Check sheet for the modelled part. Datum: model origin and axes. Units: mm. A direction names the side the tool comes from. Give positions to 0.01 mm unless a question says otherwise; leave off trailing zeros. Write each loop counter-clockwise with the first axis right and the second up, starting at its lowest first coordinate (ties: lowest second). Pieces come first, ordered by that corner, then holes. Notation, with made-up numbers: (65.5, 20.5) -> (79.5, 20.5) arc R16 cw to (79.5, 37.5) -> close; hole circle Ø9 at (75, 1). An arc over 180 degrees is marked (long way). Answer as a JSON object with one key per item and string values.
from build123d import *

# Parameters (mm, degrees)
SKETCH1_W           = 22
SKETCH1_H           = 11
BOSS_EXTRUDE1_DEPTH = 24
BOSS_EXTRUDE2_DEPTH = 4
SKETCH4_W           = 11
SKETCH4_H           = 2
BOSS_EXTRUDE3_DEPTH = 3
SKETCH5_R           = 1
CUT_EXTRUDE2_DEPTH  = 21
SKETCH3_R           = 2.25
BOSS_EXTRUDE4_DEPTH = 3


with BuildPart() as part:
    # Sketch1 → Boss-Extrude1 (new body)
    with BuildSketch(Plane(origin=(0, 0, 0), x_dir=(1, 0, 0), z_dir=(0, 1, 0))):
        Rectangle(SKETCH1_W, SKETCH1_H)
    extrude(amount=BOSS_EXTRUDE1_DEPTH)

    # Sketch2 → Boss-Extrude2 (add)
    with BuildSketch(Plane(origin=(0, 24, 0), x_dir=(1, 0, 0), z_dir=(0, 1, 0))):
        with BuildLine():
            Line((-0.5, 2.006506876), (0.376524617, 2.006506876))
            ThreePointArc((0.376524617, 2.006506876), (11, 0.006506876), (0.376524617, -1.993493124))
            Line((0.376524617, -1.993493124), (-0.5, -1.993493124))
            ThreePointArc((-0.5, -1.993493124), (-2.5, 0.006506876), (-0.5, 2.006506876))
        make_face()
    extrude(amount=BOSS_EXTRUDE2_DEPTH)

    # Sketch4 → Boss-Extrude3 (add)
    with BuildSketch(Plane.ZY.offset(11)):
        with Locations((0, 19)):
            Rectangle(SKETCH4_W, SKETCH4_H)
    boss_extrude3 = extrude(amount=BOSS_EXTRUDE3_DEPTH)

    # Sketch5 → Cut-Extrude2 (cut, through all)
    with BuildSketch(Plane(origin=(0, 20, 0), x_dir=(1, 0, 0), z_dir=(0, 1, 0))):
        with Locations((-12.5, 0)):
            Circle(SKETCH5_R)
    cut_extrude2 = extrude(amount=-CUT_EXTRUDE2_DEPTH, mode=Mode.SUBTRACT)

    # Mirror1: Boss-Extrude3, Cut-Extrude2 across plane
    add(boss_extrude3.mirror(Plane(origin=(0, 0, 0), x_dir=(0, 0, 1), z_dir=(1, 0, 0))))
    add(cut_extrude2.mirror(Plane(origin=(0, 0, 0), x_dir=(0, 0, 1), z_dir=(1, 0, 0))), mode=Mode.SUBTRACT)

    # Sketch3 → Boss-Extrude4 (add)
    with BuildSketch(Plane(origin=(0, 28, 0), x_dir=(1, 0, 0), z_dir=(0, 1, 0))):
        with Locations((5.5, 0.006506876)):
            Circle(SKETCH3_R)
    extrude(amount=BOSS_EXTRUDE4_DEPTH)


solid = part.part
1. Sectioned sample at A-A, the plane x = 12.5. Enter the section's corners in (y, z), plus the area to 3 significant figures.
Determined:
{"outline": "(18, -5.5) -> (20, -5.5) -> (20, -1) -> (18, -1) -> close; (18, 1) -> (20, 1) -> (20, 5.5) -> (18, 5.5) -> close", "area": "18.0 mm^2"}
2. Sectioned sample at C-C, the plane x = -5.25. Enter the section's corners in (y, z), plus the area to 3 significant figures.
Determined:
{"outline": "(0, -5.5) -> (24, -5.5) -> (24, 5.5) -> (0, 5.5) -> close", "area": "264 mm^2"}
3. Mould release check, pull along Z, two halves, no side actions. Record for faces 4 (the face through (12.5, 18, -1.3)), 5 (the face through (11, 26, 0)), 6 (the face through (-13.5, 19, 0)): released by +Z, released by -Z, zero draft, split by the parting line, or undercut.
Determined:
{"face 4": "zero draft", "face 5": "split by the parting line", "face 6": "undercut"}
4. Sectioned sample at B-B, the plane z = -3.75. Enter the section's corners in (x, y).
Determined:
{"outline": "(-14, 18) -> (-11, 18) -> (-11, 0) -> (11, 0) -> (11, 18) -> (14, 18) -> (14, 20) -> (11, 20) -> (11, 24) -> (9.53, 24) -> (9.53, 28) -> (1.47, 28) -> (1.47, 24) -> (-11, 24) -> (-11, 20) -> (-14, 20) -> close"}
5. Scan lines: L1, parallel to X at y = 18.6, z = 0; L2, parallel to Z at x = 12.5, y = 19.3; L3, parallel to X at y = 6, z = 1. Record each from-to range of solid material in increasing order. Write a range as [from, to].
Determined:
{"L1": "[-14, -13.5], [-11.5, 11.5], [13.5, 14]", "L2": "[-5.5, -1], [1, 5.5]", "L3": "[-11, 11]"}
6. Go/stop test with flat-tipped pins: P1, Ø1, axis at x = 0, y = 26, coming from the -Z side; P2, Ø1, axis at y = 10, z = -2.5, coming from the -X side; P3, Ø1.8, axis at x = 12.5, z = 0, coming from the +Y side; P4, Ø1, axis at x = -3.5, y = 21, coming from the -Z side. Record where each tip stops, or that it passes through.
Determined:
{"P1": "z = -2.3", "P2": "x = -11", "P3": "through", "P4": "z = -5.5"}
7. Access from +Z, -Z, +X, -X, +Y, -Y to the whole of each face (thin tool, end or side, straight path). Record for faces 1 (the face through (3, 28, 0)), 2 (the face through (-2.5, 26, 0)), 3 (the face through (0, 26, -2.007)).
Determined:
{"face 1": "+Y", "face 2": "-X, +Y", "face 3": "-Z, -X, +Y"}
8. Sectioned sample at D-D, the plane y = 11. Enter the section's corners in (x, z), plus the area to 3 significant figures.
Determined:
{"outline": "(-11, -5.5) -> (11, -5.5) -> (11, 5.5) -> (-11, 5.5) -> close", "area": "242 mm^2"}
